CAD build for the part. Positions are in the model's coordinates, mm. A direction names the side the tool comes from. Coordinates: 2 decimals unless noted, no trailing zeros. Loops run counter-clockwise (first coordinate to the right, second up) from the corner with the lowest first, then second, coordinate; pieces in that order, holes last.
1) Pin check, flat tip, straight feed: pin 1 Ø4 at (x, z) = (-30, 0) entering from +Y (3 decimals). Stop position of the tip, or through.
2) Which spindle directions (+Z, -Z, +X, -X, +Y, -Y) get a long thin tool onto all of the face, cutting with end or side? Do faces 1 (the flat face through (0, 0, -12.7)), 2 (the flat face through (-8, 3.175, 1)). Say none if no direction does.
3) Two-plate mould, pull along Z, no slides. Class faces 3 (the cylindrical face through (17.996, 0.044, 40.626)), 4 (the flat face through (35.56, 0, -1)), 5 (the flat face through (0, 0, -58.42)): +Z half, -Z half, draft (parallel to the pull), parting line (faces both ways), or undercut.
4) Saw through at A-A, the plane z = -6. Write the cut outline in (x, y) (3 decimals), and give its area (3 significant figures).
5) Saw through at C-C, the plane y = 1. Give the number of separate pieces and of enclosed holes in the cut face, and give its area (3 significant figures).
6) Saw through at B-B, the plane x = 0. Write the cut outline in (y, z) (1 decimal), and give its area (3 significant figures).
7) Wall check: line 1 along X through (y, z) = (0.5, 2); line 2 along X through (y, z) = (-2.5, -18.5); line 3 along Z through (x, y) = (-1, 1.75). Give the ranges that are in metal, low to high.
```python
from build123d import *

# Parameters (mm, degrees)
F0_R     = 1.5875
F0_W     = 6.35
F0_H     = 38.1
F1_DEPTH = 3.175
F2_DEPTH = 2.54


# Not quite as in the source:
# - a feature names something its author has since deleted; it is built from what else it names


with BuildPart() as f1:
    # F0 (on Front) → F1 (new body, symmetric)
    with BuildSketch(Plane.XZ):
        Polygon((35.56, -58.42), (35.56, 58.42), (-35.56, 58.42), (-35.56, 0), (-35.56, -58.42), align=None)
        with Locations((-17.1425342897, -39.2875)):
            Circle(F0_R, mode=Mode.SUBTRACT)
        with Locations((0, -41.656)):
            Circle(F0_R, mode=Mode.SUBTRACT)
        with BuildLine():
            ThreePointArc((-28.4118865192, 0), (-29.9993865192, -1.5875), (-31.5868865192, 0))
            ThreePointArc((-31.5868865192, 0), (-29.9993865192, 1.5875), (-28.4118865192, 0))
        make_face(mode=Mode.SUBTRACT)
        Polygon((-6.35, -12.7), (-6.35, 12.7), (0, 12.7), (6.35, 12.7), (6.35, -12.7), align=None, mode=Mode.SUBTRACT)
        with Locations((17.1425342897, -39.2875)):
            Circle(F0_R, mode=Mode.SUBTRACT)
        with Locations((15.1556345809, 0)):
            Rectangle(F0_W, F0_H, mode=Mode.SUBTRACT)
        with Locations((29.1256345809, 0)):
            Rectangle(F0_W, F0_H, mode=Mode.SUBTRACT)
        with Locations((-17.1425342897, 39.2875)):
            Circle(F0_R, mode=Mode.SUBTRACT)
        with BuildLine():
            ThreePointArc((1.5875, 41.656), (1.1225320151, 40.5334679849), (0, 40.0685))
            ThreePointArc((0, 40.0685), (-1.1225320151, 42.7785320151), (1.5875, 41.656))
        make_face(mode=Mode.SUBTRACT)
        with Locations((17.1425342897, 39.2875)):
            Circle(F0_R, mode=Mode.SUBTRACT)
    extrude(amount=F1_DEPTH, both=True)

    # F0 (on Front) → F2 (cut)
    with BuildSketch(Plane.XZ):
        with Locations((15.1556345809, 0)):
            Rectangle(F0_W, F0_H)
        with Locations((29.1256345809, 0)):
            Rectangle(F0_W, F0_H)
    extrude(amount=-F2_DEPTH, mode=Mode.SUBTRACT)


solid = f1.part
```
Data:
1. pin 1: stops at y = 3.175
2. face 1: +Y, -Y
2. face 2: +Z, -Z, +X, -X, +Y
3. face 3: undercut
3. face 4: draft
3. face 5: -Z half
4. outline: (-35.56, -3.175) - (-6.35, -3.175) - (-6.35, 3.175) - (-35.56, 3.175) - close; (6.35, -3.175) - (11.981, -3.175) - (11.981, 3.175) - (6.35, 3.175) - close; (18.331, -3.175) - (25.951, -3.175) - (25.951, 3.175) - (18.331, 3.175) - close; (32.301, -3.175) - (35.56, -3.175) - (35.56, 3.175) - (32.301, 3.175) - close
4. area: 290 mm2
5. separate pieces: 1
5. enclosed holes: 10
5. area: 7,450 mm2
6. outline: (-3.2, -58.4) - (3.2, -58.4) - (3.2, -43.2) - (-3.2, -43.2) - close; (-3.2, -40.1) - (3.2, -40.1) - (3.2, -12.7) - (-3.2, -12.7) - close; (-3.2, 12.7) - (3.2, 12.7) - (3.2, 40.1) - (-3.2, 40.1) - close; (-3.2, 43.2) - (3.2, 43.2) - (3.2, 58.4) - (-3.2, 58.4) - close
6. area: 540 mm2
7. line 1: x = -35.56 to -6.35, 6.35 to 11.98, 18.33 to 25.95, 32.3 to 35.56
7. line 2: x = -35.56 to 11.98, 18.33 to 25.95, 32.3 to 35.56
7. line 3: z = -58.42 to -42.89, -40.42 to -12.7, 12.7 to 40.42, 42.89 to 58.42
